Input: part model. Units: mm. Frame: model coordinates. Face numbers are marked on the shaded views. A direction names the side the tool comes from. Coordinates: 2 decimals unless noted, no trailing zeros. Order: outer loops, then holes, each group sorted by start corner. A loop starts at its lowest first (then second) coordinate and runs counter-clockwise, first axis right, second up. Notation, with made-up numbers: (36.25, -19.5) -> (43.25, -19.5) arc R24 cw to (43.25, -0.5) -> close; hole circle Ø7 at (63.5, 18.5). An arc over 180 degrees is marked (long way). One line per question, with ' | ' between items.
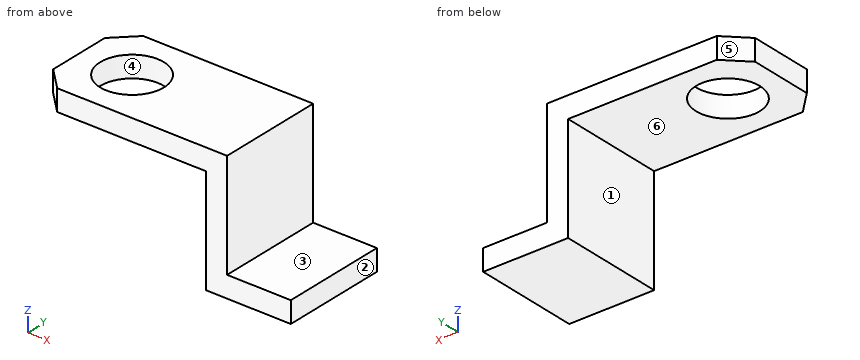
```python
from build123d import *

# Parameters (mm, degrees)
F0_W      = 16
F0_H      = 10
F1_DEPTH  = 2
F2_SIZE   = 2
F7_D      = 6
F8_W      = 10
F8_H      = 2
F8_H_2    = 10
F9_DEPTH  = 2
F10_W     = 10
F10_H     = 2
F11_DEPTH = 6


with BuildPart() as f1:
    # F0 (on Top) → F1 (new body)
    with BuildSketch(Plane.XY):
        with Locations((8, -5)):
            Rectangle(F0_W, F0_H)
    extrude(amount=F1_DEPTH)

    # F2
    f2_edges = [f1.edges().sort_by_distance(p)[0] for p in [
        (0, -10, 1),
        (0, 0, 1),
    ]]
    chamfer(f2_edges, length=F2_SIZE)

    # F7 (through all)
    with Locations(Plane.XY.offset(2)):
        with Locations((5, -5)):
            Hole(F7_D / 2)

    # F8 (on face) → F9 (join)
    with BuildSketch(Plane.YZ.offset(16)):
        with Locations((-5, 1)):
            Rectangle(F8_W, F8_H)
        with Locations((-5, -5)):
            Rectangle(F8_W, F8_H_2)
    extrude(amount=F9_DEPTH)

    # F10 (on face) → F11 (join)
    with BuildSketch(Plane.YZ.offset(18)):
        with Locations((-5, -9)):
            Rectangle(F10_W, F10_H)
    extrude(amount=F11_DEPTH)


solid = f1.part
```
1. Cut plane A-A, the plane y = -5. Return loops of the section in (x, z), and give its area (3 significant figures).
Recorded:
outline: (0, 0) -> (2, 0) -> (2, 2) -> (0, 2) -> close; (8, 0) -> (16, 0) -> (16, -10) -> (24, -10) -> (24, -8) -> (18, -8) -> (18, 2) -> (8, 2) -> close | area: 56.0 mm^2
2. Mould query, pull axis Y, two halves, no side actions, for the marked faces 4, 5 and 6. Classes: released by +Y, released by -Y, zero draft, split by the parting line, or undercut.
Recorded:
face 4: undercut | face 5: released by +Y | face 6: zero draft
3. Ray query, line 1 (Y direction, x = 5, z = 0.95); line 2 (X direction, y = -8.25, z = -3.75); line 3 (Z direction, x = 1.5, y = -4.75). Return the intervals inside material, ascending. Write a range as [from, to].
Recorded:
line 1: y = [-10, -8], [-2, 0] | line 2: x = [16, 18] | line 3: z = [0, 2]
4. Cut plane D-D, the plane z = -5.75. Return loops of the section in (x, y), and give its area (3 significant figures).
Recorded:
outline: (16, -10) -> (18, -10) -> (18, 0) -> (16, 0) -> close | area: 20.0 mm^2
5. Cut plane C-C, the plane y = -8.75. Return loops of the section in (x, z), and give its area (3 significant figures).
Recorded:
outline: (0.75, 0) -> (16, 0) -> (16, -10) -> (24, -10) -> (24, -8) -> (18, -8) -> (18, 2) -> (0.75, 2) -> close | area: 66.5 mm^2
6. Access query for the marked faces 1, 2 and 3. Directions: +Z, -Z, +X, -X, +Y, -Y. A direction counts if a zero-diameter tool reaches every point of the face in a straight line with its end or side. Return the directions, or none.
Recorded:
face 1: -Z, -X, +Y, -Y | face 2: +Z, -Z, +X, +Y, -Y | face 3: +Z, +X, +Y, -Y
7. Pin query (flat end, axial travel): pin 1 Ø6 at (x, y) = (7.5, -6) entering from -Z; pin 2 Ø1.5 at (y, z) = (-7, -7) entering from -X; pin 3 Ø1.8 at (x, y) = (19.5, -3) entering from +Z; pin 4 Ø3 at (x, y) = (6.5, -7) entering from +Z. Return the tip coordinate at first contact, or that it passes through.
Recorded:
pin 1: stops at z = 0 | pin 2: stops at x = 16 | pin 3: stops at z = -8 | pin 4: stops at z = 2
8. Cut plane B-B, the plane x = 5. Return loops of the section in (y, z), and give its area (3 significant figures).
Recorded:
outline: (-10, 0) -> (-8, 0) -> (-8, 2) -> (-10, 2) -> close; (-2, 0) -> (0, 0) -> (0, 2) -> (-2, 2) -> close | area: 8.00 mm^2
